from build123d import *

# Parameters (mm, degrees)
F3_DEPTH = 25


with BuildPart() as f1:
    # F0 (on Front) → F1 (revolve)
    with BuildSketch(Plane.XZ):
        with BuildLine():
            Line((-96, 54.58075), (-96, 8.58075))
            Line((-96, 8.58075), (96, 8.58075))
            Line((96, 8.58075), (96, 54.58075))
            Line((96, 54.58075), (60, 54.58075))
            Line((60, 54.58075), (60, 205))
            ThreePointArc((60, 205), (0, 175), (-60, 205))
            Line((-60, 205), (-60, 54.58075))
            Line((-60, 54.58075), (-96, 54.58075))
        make_face()
        with BuildLine():
            ThreePointArc((75, 250), (-23.717082, 321.151247), (-60, 205))
            ThreePointArc((-60, 205), (0, 175), (60, 205))
            ThreePointArc((60, 205), (71.151247, 226.282918), (75, 250))
        make_face()
    revolve(axis=Axis((0, 0, 0), (1, 0, 0)))

    # F2 (on face) → F3 (join)
    with BuildSketch(Plane(origin=(-60, 0, 0), x_dir=(0, -1, 0), z_dir=(-1, 0, 0))):
        with BuildLine():
            ThreePointArc((-54.100605, 185.262313), (-60.432679, 179.731135), (-60.307153, 171.324392))
            Line((-60.307153, 171.324392), (-12.55207, 72.159939))
            ThreePointArc((-12.55207, 72.159939), (-8.665392, 67.910717), (-3.079813, 66.509481))
            ThreePointArc((-3.079813, 66.509481), (0, 66.58075), (3.079813, 66.509481))
            ThreePointArc((3.079813, 66.509481), (8.665392, 67.910717), (12.55207, 72.159939))
            Line((12.55207, 72.159939), (60.307153, 171.324392))
            ThreePointArc((60.307153, 171.324392), (60.432679, 179.731135), (54.100605, 185.262313))
            ThreePointArc((54.100605, 185.262313), (0, 193), (-54.100605, 185.262313))
        make_face()
    extrude(amount=-F3_DEPTH)


solid = f1.part
Model file for the job. Use its own axes, mm. A direction names the side the tool comes from. Give positions to 0.01 mm unless a question says otherwise; leave off trailing zeros. Loops run counter-clockwise (first coordinate to the right, second up) from the corner with the lowest first, then second, coordinate; pieces in that order, holes last. Notation, with made-up numbers: (83.5, 9) -> (134.5, 9) arc R25 ccw to (134.5, 28) -> close; hole circle Ø11 at (-35, 74). An arc over 180 degrees is marked (long way). Use a Markdown table: item, result. Add a question column.
(1) Slice it at A-A on y = 0. List the corners of the cut face in (x, z).
(2) Wall check: line 1 along Y through (x, z) = (-1, 0); line 2 along X through (y, z) = (139, -137.5); line 3 along Z through (x, y) = (-33, 0). Give the ranges that are in metal, low to high.
(3) Drop flat-ended pins along their axis: pin 1 Ø1.5 at (x, y) = (-26.5, 33.5) entering from +Z; pin 2 Ø12 at (x, z) = (-42.5, 83.5) entering from +Y; pin 3 Ø6 at (y, z) = (244, -188.5) entering from +X. Give the stop position or say it passes through.
(4) Slice it at D-D on x = 20.5. List the corners of the cut face in (y, z), and give its area (3 significant figures).
(5) Mould opens along Z. For faces 1 (the flat face through (-96, 11, -1)), 2 (the cylindrical face through (77.75, -16.39, 52.06)) say: +Z half, -Z half, draft (parallel to the pull), parting line (faces both ways), or undercut.
(6) Tool access for faces 3 (the cylindrical face through (1.344, -8.508, -1.117)), 4 (the flat face through (60, 43, -43)), 5 (the cylindrical face through (-78.25, -16.39, 52.06)): list every direction of +Z, -Z, +X, -X, +Y, -Y with a clear straight run to the whole face (end or side of a thin tool).
(7) Slice it at C-C on x = -27.5. List the corners of the cut face in (y, z), and give its area (3 significant figures).
Filled sheet:
| question | item | result |
|---|---|---|
| 1 | outline | (-96, -54.58) -> (-60, -54.58) -> (-60, -205) arc R75 ccw (long way) to (75, -250) arc R75 ccw to (60, -205) -> (60, -54.58) -> (96, -54.58) -> (96, -8.58) -> (-96, -8.58) -> close; (-96, 8.58) -> (96, 8.58) -> (96, 54.58) -> (60, 54.58) -> (60, 205) arc R75 ccw to (75, 250) arc R75 ccw (long way) to (-60, 205) -> (-60, 54.58) -> (-96, 54.58) -> close |
| 2 | line 1 | -324.99 to -8.58, 8.58 to 324.99 |
| 2 | line 2 | -60 to 60 |
| 2 | line 3 | -317.35 to -8.58, 8.58 to 317.35 |
| 3 | pin 1 | z = 318.7 |
| 3 | pin 2 | y = 304.63 |
| 3 | pin 3 | x = 50.63 |
| 4 | outline | circle Ø644.29 at (0, 0); hole circle Ø17.16 at (0, 0) |
| 4 | area | 326,000 mm2 |
| 5 | face 1 | draft |
| 5 | face 2 | undercut |
| 6 | face 3 | +X, -X |
| 6 | face 4 | +X |
| 6 | face 5 | -X |
| 7 | outline | circle Ø639.55 at (0, 0); hole circle Ø17.16 at (0, 0) |
| 7 | area | 321,000 mm2 |
